For this review, take the finished solid that the model builds, in its own axes (mm). Round coordinates to 2 decimals unless told otherwise and drop trailing zeros. Order: outer loops, then holes, each group sorted by start corner. A loop starts at its lowest first (then second) coordinate and runs counter-clockwise, first axis right, second up. Notation, with made-up numbers: M 84.5,19.25 L 110.5,19.25 A26 ccw 110.5,54.25 Z; hole C -16.75,-34 d7. An arc over 180 degrees is marked long. Put each result on its own line as item: value.
from build123d import *

# Parameters (mm, degrees)
F0_W     = 25.4
F0_H     = 50.8
F1_DEPTH = 6.35
F2_R     = 3.175
F3_DEPTH = 25.4
F4_R     = 3.81


with BuildPart() as f1:
    # F0 (on Top) → F1 (new body)
    with BuildSketch(Plane.XY):
        Rectangle(F0_W, F0_H)
    extrude(amount=F1_DEPTH)

    # F2 (on face) → F3 (cut)
    with BuildSketch(Plane.XY.offset(6.35)):
        with Locations((-6.35, 19.05)):
            Circle(F2_R)
    extrude(amount=-F3_DEPTH, mode=Mode.SUBTRACT)

    # F4
    f4_edges = [f1.edges().sort_by_distance(p)[0] for p in [
        (-12.7, 25.4, 3.175),
        (12.7, 25.4, 3.175),
        (-12.7, -25.4, 3.175),
        (12.7, -25.4, 3.175),
    ]]
    fillet(f4_edges, radius=F4_R)


solid = f1.part
(1) Add section C-C on y = 19.05. Give the boundary of the cut face in (x, z) (3 decimals), then the cut area to 3 significant figures.
A:
outline: M -12.7,0 L -9.525,0 L -9.525,6.35 L -12.7,6.35 Z; M -3.175,0 L 12.7,0 L 12.7,6.35 L -3.175,6.35 Z
area: 121 mm2
(2) To check wall thickness, follow L1, parallel to Y at x = -6.35, z = 4.25 (3 decimals); L2, parallel to Y at x = -4, z = 0.75; L3, parallel to X at y = 23, z = 4.75. State the ranges of each line that lie inside material, in increasing order.
A:
L1: y = -25.4 to 15.875, 22.225 to 25.4
L2: y = -25.4 to 16.92, 21.18 to 25.4
L3: x = -12.43 to 12.43
(3) Add section A-A on x = -6.35. Give the boundary of the cut face in (y, z) (3 decimals).
A:
outline: M -25.4,0 L 15.875,0 L 15.875,6.35 L -25.4,6.35 Z; M 22.225,0 L 25.4,0 L 25.4,6.35 L 22.225,6.35 Z
(4) Add section B-B on z = 2.75. Give the boundary of the cut face in (x, y) (3 decimals), then the cut area to 3 significant figures.
A:
outline: M -12.7,-21.59 A3.81 ccw -8.89,-25.4 L 8.89,-25.4 A3.81 ccw 12.7,-21.59 L 12.7,21.59 A3.81 ccw 8.89,25.4 L -8.89,25.4 A3.81 ccw -12.7,21.59 Z; hole C -6.35,19.05 d6.35
area: 1,250 mm2
(5) Draft analysis for pull direction Y (two halves, no side actions). For faces 1 (the face through (-7.04, 15.95, 3.22)), 2 (the face through (11.554, 24.314, 3.219)), 3 (the face through (-11.614, -24.254, 3.219)), state which applies: released by +Y, released by -Y, zero draft, split by the parting line, or undercut.
A:
face 1: undercut
face 2: released by +Y
face 3: released by -Y
